Build history of the part. All positions in model axes, mm. A direction names the side the tool comes from. Round coordinates to 2 decimals unless told otherwise and drop trailing zeros. Order: outer loops, then holes, each group sorted by start corner. A loop starts at its lowest first (then second) coordinate and runs counter-clockwise, first axis right, second up. Notation, with made-up numbers: M 21.5,37.25 L 68.5,37.25 A8 ccw 68.5,52.25 Z; hole C 54.5,43.25 d9. An arc over 180 degrees is marked long. One line per item, written item: value. Start each with the question number.
Item 1: Band-saw the part on A-A, the plane y = 54.25. Write the cut outline in (x, z).
Item 2: Band-saw the part on B-B, the plane z = 15. Write the cut outline in (x, y), then the cut area to 3 significant figures.
Item 3: Band-saw the part on C-C, the plane y = 62.75. Write the cut outline in (x, z), then the cut area to 3 significant figures.
Item 4: Probe L1, parallel to X at y = 55.25, z = 14; L2, parallel to Z at x = 120.5, y = 61; L3, parallel to Y at x = 168, z = 9.75. List the from-to ranges inside material, lowest first.
Item 5: Tool access for faces 5 (the flat face through (142, 65.144, 6)), 6 (the flat face through (167.901, 57, 17)), 7 (the flat face through (142, 56.254, 4)): list every direction of +Z, -Z, +X, -X, +Y, -Y with a clear straight run to the whole face (end or side of a thin tool).
Item 6: Pin check, flat tips, straight feed: pin 1 (2.5 mm diameter, centred on x = 144, y = 62.5, fed in from +Z); pin 2 (6 mm diameter, centred on x = 132, z = 6.5, fed in from -Y); pin 3 (12 mm diameter, centred on x = 152.5, y = 49, fed in from -Z). Stop position of each tip, or through.
Item 7: Two-plate mould, pull along X, no slides. Class faces 1 (the flat face through (111.95, 49.815, 17.089)), 2 (the flat face through (106.941, 59, 14)), 3 (the flat face through (178.061, 59, 14)), 4 (the flat face through (117.101, 57, 17)): +X half, -X half, draft (parallel to the pull), parting line (faces both ways), or undercut.
```python
from build123d import *

# Parameters (mm, degrees)
SKETCH1_W           = 71.12
SKETCH1_H           = 8.89
BOSS_EXTRUDE1_DEPTH = 6.35
SKETCH5_W           = 10.16
SKETCH5_H           = 8.89
BOSS_EXTRUDE5_DEPTH = 17
SKETCH6_W           = 10.16
SKETCH6_H           = 12.7
BOSS_EXTRUDE6_DEPTH = 12.7
CHAMFER3_SIZE       = 12.7


with BuildPart() as part:
    # Sketch1 → Boss-Extrude1 (new body)
    with BuildSketch(Plane.XY):
        with Locations((142.501032585, 60.698661386)):
            Rectangle(SKETCH1_W, SKETCH1_H)
    extrude(amount=BOSS_EXTRUDE1_DEPTH)

    # Sketch5 → Boss-Extrude5 (add)
    with BuildSketch(Plane.XY.offset(6.35)):
        with Locations((112.021032585, 60.698661386)):
            Rectangle(SKETCH5_W, SKETCH5_H)
        with Locations((172.981032585, 60.698661386)):
            Rectangle(SKETCH5_W, SKETCH5_H)
    extrude(amount=BOSS_EXTRUDE5_DEPTH)

    # Sketch6 → Boss-Extrude6 (add)
    with BuildSketch(Plane.XZ.offset(-56.253661386)):
        with Locations((172.981032585, 17)):
            Rectangle(SKETCH6_W, SKETCH6_H)
        with Locations((112.021032585, 17)):
            Rectangle(SKETCH6_W, SKETCH6_H)
    extrude(amount=BOSS_EXTRUDE6_DEPTH)

    # Chamfer3
    chamfer3_edges = [part.edges().sort_by_distance(p)[0] for p in [
        (112.021032585, 43.553661386, 10.65),
        (172.981032585, 43.553661386, 10.65),
    ]]
    chamfer(chamfer3_edges, length=CHAMFER3_SIZE - 0.0001)  # a hair under: the kernel refuses the full size


solid = part.part
```
Output:
1. outline: M 106.94,12.65 L 117.1,12.65 L 117.1,23.35 L 106.94,23.35 Z; M 167.9,12.65 L 178.06,12.65 L 178.06,23.35 L 167.9,23.35 Z
2. outline: M 106.94,51.9 L 117.1,51.9 L 117.1,65.14 L 106.94,65.14 Z; M 167.9,51.9 L 178.06,51.9 L 178.06,65.14 L 167.9,65.14 Z
2. area: 269 mm²
3. outline: M 106.94,0 L 178.06,0 L 178.06,23.35 L 167.9,23.35 L 167.9,6.35 L 117.1,6.35 L 117.1,23.35 L 106.94,23.35 Z
3. area: 797 mm²
4. L1: x = 106.94 to 117.1, 167.9 to 178.06
4. L2: z = 0 to 6.35
4. L3: y = 56.25 to 65.14
5. face 5: +Z, -Z, +X, -X, +Y
5. face 6: +Z, +Y, -Y
5. face 7: -Z, +X, -X, -Y
6. pin 1: stops at z = 6.35
6. pin 2: stops at y = 56.25
6. pin 3: passes through
7. face 1: draft
7. face 2: -X half
7. face 3: +X half
7. face 4: undercut
